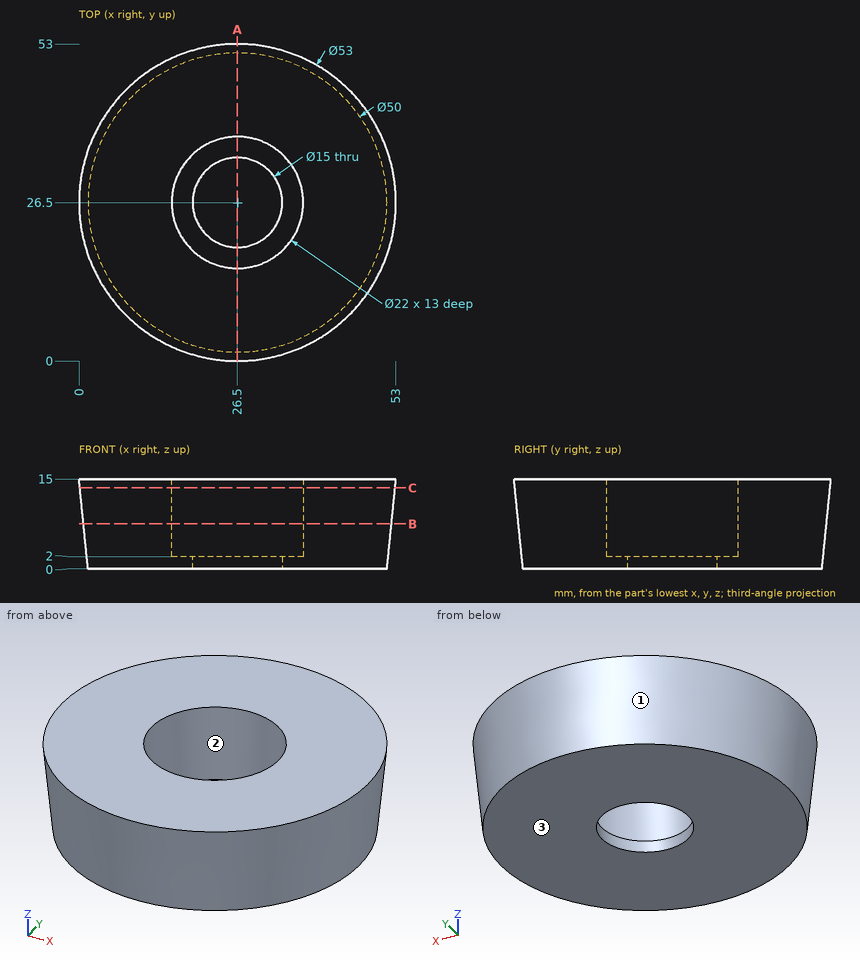
Drawing for the job (mm, zero at the part's lowest x, y, z). Round coordinates to 2 decimals unless told otherwise and drop trailing zeros. Loops run counter-clockwise (first coordinate to the right, second up) from the corner with the lowest first, then second, coordinate; pieces in that order, holes last. Notation, with made-up numbers: M 25.25,26.25 L 30.25,26.25 A14 cw 30.25,48.25 Z; hole C -13.75,72.25 d2. An arc over 180 degrees is marked long. Use a Markdown table: item, result. Add a question column.
(1) Cut at B-B (z = 7.5). Give the cut face in (x, y), and give its area (3 significant figures).
(2) Drill centre lines: line 1 (Y direction, x = 26.5, z = 7.25) (3 decimals); line 2 (X direction, y = 31.5, z = 9); line 3 (X direction, y = 27, z = 4.5). Where is each one in solid material? Low to high.
(3) Cut at C-C (z = 13.5). Give the cut face in (x, y).
(4) Pull direction X, two halves, no side cores. Call the marked faces 1, 2 and 3: +X half, -X half, draft (parallel to the pull), parting line (faces both ways), or undercut.
(5) Flat gauge pins, fed straight in: pin 1 (1 mm diameter, centred on x = 18, y = 29, fed in from +Z); pin 2 (2 mm diameter, centred on y = 43, z = 4, fed in from -X); pin 3 (3 mm diameter, centred on x = 36.5, z = 3.5, fed in from +Y). Where does each tip first touch, or does it go through?
(6) Cut at A-A (x = 26.5). Give the cut face in (y, z), and give its area (4 significant figures).
Geometry says:
| question | item | result |
|---|---|---|
| 1 | outline | C 26.5,26.5 d51.5; hole C 26.5,26.5 d22 |
| 1 | area | 1,700 mm² |
| 2 | line 1 | y = 0.775 to 15.5, 37.5 to 52.225 |
| 2 | line 2 | x = 1.09 to 16.7, 36.3 to 51.91 |
| 2 | line 3 | x = 1.05 to 15.51, 37.49 to 51.95 |
| 3 | outline | C 26.5,26.5 d52.7; hole C 26.5,26.5 d22 |
| 4 | face 1 | parting line |
| 4 | face 2 | undercut |
| 4 | face 3 | draft |
| 5 | pin 1 | stops at z = 2 |
| 5 | pin 2 | stops at x = 6.37 |
| 5 | pin 3 | stops at y = 50.41 |
| 6 | outline | M 0,15 L 1.5,0 L 19,0 L 19,2 L 15.5,2 L 15.5,15 Z; M 34,0 L 51.5,0 L 53,15 L 37.5,15 L 37.5,2 L 34,2 Z |
| 6 | area | 456.5 mm² |
